Autodesk Fusion 360 part; units mm, degrees
sketch "Hex Polygon" plane through (0, 0, 0) normal (0, 0, 1) x (1, 0, 0) in component "Hex Nut"
  line L0 (-5.7735, 10) -> (-11.547, 0)
  line L1 (-11.547, 0) -> (-5.7735, -10)
  line L2 (-5.7735, -10) -> (5.7735, -10)
  line L3 (5.7735, -10) -> (11.547, 0)
  line L4 (11.547, 0) -> (5.7735, 10)
  line L5 (5.7735, 10) -> (-5.7735, 10)
  dimension "d1" = 10
extrude "Extrude1" add sketch "Hex Polygon" along normal blind 10 in component "Hex Nut"
sketch "Chamfer Cutout" plane through (0, 0, 0) normal (0, 1, 0) x (1, 0, 0) in component "Hex Nut"
  line L0 (11.547, -10) -> (10.047, -10)
  line L1 (10.047, -10) -> (11.547, -8.5)
  line L2 (11.547, -8.5) -> (11.547, -10)
  point P0 (11.547, -10)
  dimension "d4" = 1.5
revolve "Revolve1" cut sketch "Chamfer Cutout" angle 360 about axis through (0, 0, 1.75) along (0, 0, 1) in component "Hex Nut"
hole "Hole1" at (-0.7219, 0.9887, 10) direction (0, 0, -1) diameter 11.035 end through all countersink diameter 14 countersink angle 90 in component "Hex Nut"
ref_plane "WorkPlane1" through (0, 0, 5) normal (0, 0, 1) x (1, 0, 0) in component "Hex Nut"
mirror "Mirror1" about plane through (0, 0, 5) normal (0, 0, 1) of "Extrude1", "Revolve1" in component "Hex Nut"
component "Hex Nut" placed x (1, 0, 0) y (0, 1, 0) z (0, 0, 1) at (0, 0, 0)
The listing builds one solid part. Answer for the finished solid, in the listing's coordinates (mm). Give positions to 0.01 mm unless a question says otherwise; leave off trailing zeros. Loops run counter-clockwise (first coordinate to the right, second up) from the corner with the lowest first, then second, coordinate; pieces in that order, holes last. Notation, with made-up numbers: M 44.5,76.5 L 57.5,76.5 A26 ccw 57.5,103.5 Z; hole C 33.5,23.25 d2. An arc over 180 degrees is marked long. Answer as CSV lines item,"result".
Item 1: The part is cut by section C-C (x = 8.75). Give the vertices of the cut face in (y, z), and give its area (3 significant figures).
Values follow:
outline,"M -4.84,0 L 4.84,0 L 4.84,10 L -4.84,10 Z"
area,"96.9 mm^2"
Item 2: The part is cut by section B-B (y = 4.75). Give the vertices of the cut face in (x, z), and give its area (3 significant figures).
Values follow:
outline,"M -8.8,0 L 8.8,0 L 8.8,10 L -8.8,10 Z"
area,"176 mm^2"
Item 3: The part is cut by section A-A (z = 8.75). Give the vertices of the cut face in (x, y), and give its area (3 significant figures).
Values follow:
outline,"M -11.55,0 L -5.77,-10 L 5.77,-10 L 11.55,0 L 5.77,10 L -5.77,10 Z"
area,"346 mm^2"
Item 4: Given pin 1 Ø6 at (y, z) = (-5.5, 7) entering from -X; pin 2 Ø5 at (y, z) = (-6.5, 5.5) entering from -X, each flat-ended and moving along its own axis, determine where each tip first touches the part or whether it passes through.
Values follow:
pin 1,"stops at x = -10.1"
pin 2,"stops at x = -9.24"
Item 5: Straight lines are drawn through the part: line 1 along X through (y, z) = (-1.75, 1); line 2 along X through (y, z) = (-7.25, 1.25); line 3 along Y through (x, z) = (-7.75, 3.75). For each, find the intervals that lie inside material, in ascending order. Write a range as [from, to].
Values follow:
line 1,"x = [-10.54, 10.54]"
line 2,"x = [-7.36, 7.36]"
line 3,"y = [-6.58, 6.58]"
